Answer from the drawing. Dimensions are ordinates in mm from the lowest x, y and z of the part. A direction names the side the tool comes from. Give positions to 0.01 mm unless a question says otherwise; leave off trailing zeros. Order: outer loops, then holes, each group sorted by start corner. A loop starts at its lowest first (then second) coordinate and runs counter-clockwise, first axis right, second up.
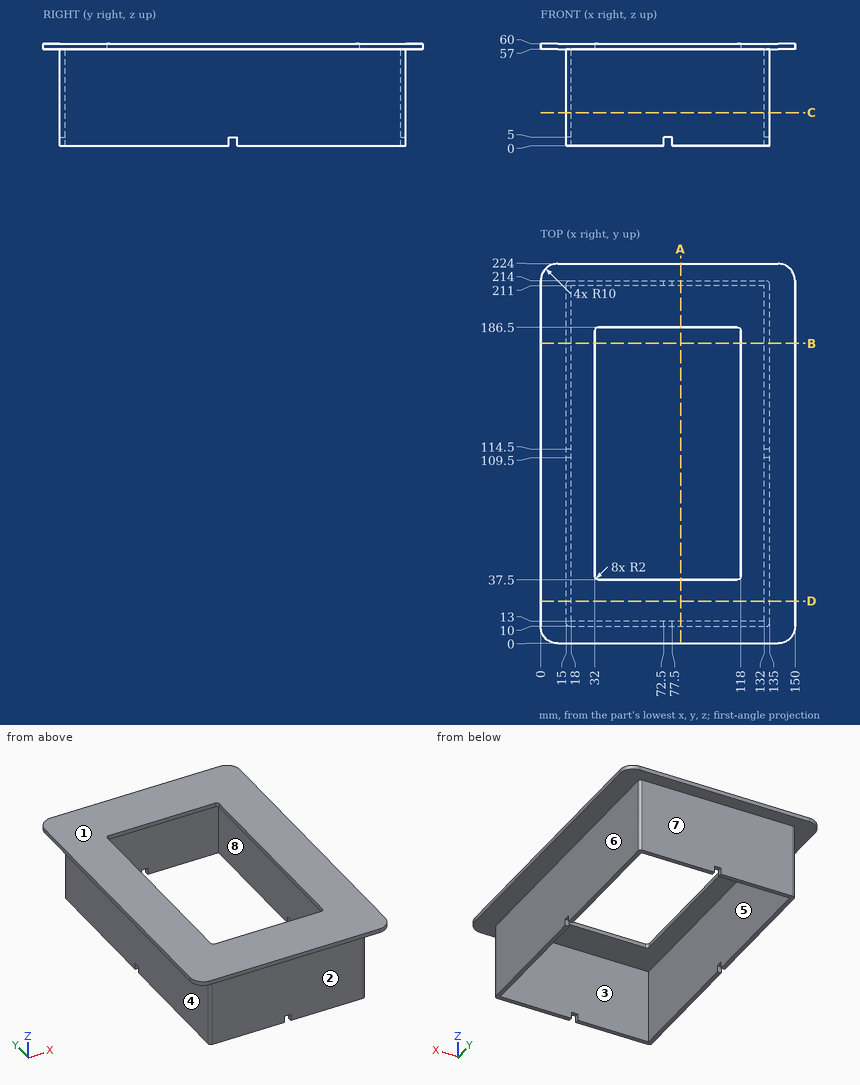
1. The part is cut by section D-D (y = 25). Write down the section's boundary in (x, z), then the cut area to 3 significant figures.
Findings below:
outline: (0, 57) - (15, 57) - (15, 0) - (18, 0) - (18, 57) - (132, 57) - (132, 0) - (135, 0) - (135, 57) - (150, 57) - (150, 60) - (0, 60) - close
area: 792 mm2
2. Given P1, Ø12, axis at x = 37, z = 43, coming from the -Y side; P2, Ø1, axis at x = 129.5, y = 81, coming from the -Z side; P3, Ø17, axis at y = 108.5, z = 30.5, coming from the -X side, each flat-ended and moving along its own axis, determine where each tip first touches the part or whether it passes through.
Findings below:
P1: stops at y = 10
P2: stops at z = 57
P3: stops at x = 15
3. The part is cut by section B-B (y = 177). Write down the section's boundary in (x, z).
Findings below:
outline: (0, 57) - (15, 57) - (15, 0) - (18, 0) - (18, 57) - (32, 57) - (32, 60) - (0, 60) - close; (118, 57) - (132, 57) - (132, 0) - (135, 0) - (135, 57) - (150, 57) - (150, 60) - (118, 60) - close
4. The part is cut by section C-C (z = 19.5). Write down the section's boundary in (x, y), then the cut area to 3 significant figures.
Findings below:
outline: (15, 12) arc R2 ccw to (17, 10) - (133, 10) arc R2 ccw to (135, 12) - (135, 212) arc R2 ccw to (133, 214) - (17, 214) arc R2 ccw to (15, 212) - close; hole (18, 13) - (132, 13) - (132, 211) - (18, 211) - close
area: 1,900 mm2
5. Which of the six approach directions +Z, -Z, +X, -X, +Y, -Y give full straight-line access (tool end or side, diameter ignored) to the marked faces 1, 2, 3 and 4?
Findings below:
face 1: +Z, +X, -X, +Y, -Y
face 2: -Z, +X, -X, -Y
face 3: -Z
face 4: -Z, -X, +Y, -Y
6. The mould has two halves that part along Y. Classify the marked faces 5, 6, 7 and 8: pulls with the +Y half, pulls with the -Y half, needs draft (parallel to the pull), parting line crosses it, or undercut.
Findings below:
face 5: undercut
face 6: needs draft
face 7: pulls with the +Y half
face 8: undercut
7. The part is cut by section A-A (x = 82.5). Write down the section's boundary in (y, z), then the cut area to 3 significant figures.
Findings below:
outline: (0, 57) - (10, 57) - (10, 0) - (13, 0) - (13, 57) - (37.5, 57) - (37.5, 60) - (0, 60) - close; (186.5, 57) - (211, 57) - (211, 0) - (214, 0) - (214, 57) - (224, 57) - (224, 60) - (186.5, 60) - close
area: 567 mm2
8. Straight lines are drawn through the part: probe 1 along Y at (x, z) = (62, 11); probe 2 along X at (y, z) = (14.5, 38); probe 3 along Z at (x, y) = (137, 124). For each, find the intervals that lie inside material, in ascending order.
Findings below:
probe 1: y = 10 to 13, 211 to 214
probe 2: x = 15 to 18, 132 to 135
probe 3: z = 57 to 60
